The model under review builds one solid part; all positions refer to its coordinate system, in mm. A direction names the side the tool comes from. Give positions to 0.01 mm unless a question says otherwise; leave off trailing zeros. Order: outer loops, then holes, each group sorted by start corner. A loop starts at its lowest first (then second) coordinate and runs counter-clockwise, first axis right, second up. Notation, with made-up numbers: (-11, -39) - (17, -39) arc R21 cw to (17, -5) - close; hole circle Ø6 at (32.5, 41). An arc over 180 degrees is marked (long way). Use a Markdown table: item, result. Add a question column.
```python
from build123d import *

# Parameters (mm, degrees)
SKETCH1_W           = 88.9
SKETCH1_H           = 25.4
SKETCH1_R           = 2.25
BOSS_EXTRUDE1_DEPTH = 3.175
SKETCH2_W           = 88.9
SKETCH2_H           = 28.575
SKETCH2_R           = 2.25
BOSS_EXTRUDE2_DEPTH = 3.175
FILLET1_R           = 1.5875
BOSS_EXTRUDE3_DEPTH = 19.05
SKETCH5_R           = 2.25
CUT_EXTRUDE1_DEPTH  = 100
FILLET2_R           = 6.35
BOSS_EXTRUDE4_START = 5
SKETCH6_R           = 3.175
SKETCH6_R_2         = 2.25
BOSS_EXTRUDE4_DEPTH = 5
FILLET3_R           = 2
FILLET4_R           = 6
FILLET5_R           = 2


with BuildPart() as part:
    # Sketch1 → Boss-Extrude1 (new body)
    with BuildSketch(Plane.XY):
        Rectangle(SKETCH1_W, SKETCH1_H)
        Circle(SKETCH1_R, mode=Mode.SUBTRACT)
        with Locations((-38.1, 0)):
            Circle(SKETCH1_R, mode=Mode.SUBTRACT)
        with Locations((38.1, 0)):
            Circle(SKETCH1_R, mode=Mode.SUBTRACT)
    extrude(amount=BOSS_EXTRUDE1_DEPTH)

    # Sketch2 → Boss-Extrude2 (add)
    with BuildSketch(Plane(origin=(0, 12.7, 0), x_dir=(1, 0, 0), z_dir=(0, 1, 0))):
        with Locations((0, 11.1125)):
            Rectangle(SKETCH2_W, SKETCH2_H)
        with Locations(Location((0, 12.7, 0), (0, 0, 180))):
            Circle(SKETCH2_R, mode=Mode.SUBTRACT)
        with Locations(Location((-38.1, 12.7, 0), (0, 0, 180))):
            Circle(SKETCH2_R, mode=Mode.SUBTRACT)
        with Locations(Location((38.1, 12.7, 0), (0, 0, 180))):
            Circle(SKETCH2_R, mode=Mode.SUBTRACT)
    extrude(amount=BOSS_EXTRUDE2_DEPTH)

    # Fillet1
    fillet1_edges = [part.edges().sort_by_distance(p)[0] for p in [
        (0, 15.875, 3.175),
    ]]
    fillet(fillet1_edges, radius=FILLET1_R)

    # Sketch4 → Boss-Extrude3 (add)
    with BuildSketch(Plane(origin=(0, 15.875, 0), x_dir=(1, 0, 0), z_dir=(0, 1, 0))):
        Polygon((-11, 12.7), (-11, 25.4), (-17.35, 25.4), (-17.35, 12.7), (-17.35, -1.5875), (-11, -1.5875), align=None)
        Polygon((11, 25.4), (11, 12.7), (11, -1.5875), (17.35, -1.5875), (17.35, 12.7), (17.35, 25.4), align=None)
    extrude(amount=BOSS_EXTRUDE3_DEPTH)

    # Sketch5 → Cut-Extrude1 (cut)
    with BuildSketch(Plane(origin=(17.35, 0, 0), x_dir=(0, 0, -1), z_dir=(1, 0, 0))):
        with Locations(Location((11.90625, 28.575, 0), (0, 0, 90))):
            Circle(SKETCH5_R)
    extrude(amount=-CUT_EXTRUDE1_DEPTH, mode=Mode.SUBTRACT)

    # Fillet2
    fillet2_edges = [part.edges().sort_by_distance(p)[0] for p in [
        (-14.175, 34.925, -25.4),
        (-14.175, 34.925, 1.5875),
        (14.175, 34.925, -25.4),
        (14.175, 34.925, 1.5875),
    ]]
    fillet(fillet2_edges, radius=FILLET2_R)

    # Sketch6 → Boss-Extrude4 (add)
    with BuildSketch(Plane(origin=(-11, 0, 0), x_dir=(0, 0, -1), z_dir=(1, 0, 0)).offset(BOSS_EXTRUDE4_START)):
        with Locations((11.90625, 28.575)):
            Circle(SKETCH6_R)
        with Locations(Location((11.90625, 28.575, 0), (0, 0, 90))):
            Circle(SKETCH6_R_2, mode=Mode.SUBTRACT)
    extrude(amount=-BOSS_EXTRUDE4_DEPTH)

    # Fillet3
    fillet3_edges = [part.edges().sort_by_distance(p)[0] for p in [
        (-11, 28.575, -8.73125),
    ]]
    fillet(fillet3_edges, radius=FILLET3_R)

    # Mirror2: part across plane


with BuildPart() as part_1:
    add(part.part)
    add(part.part.mirror(Plane(origin=(0, 0, 0), x_dir=(0, 0, 1), z_dir=(1, 0, 0))))

    # Fillet4
    # the kernel refuses this fillet: 6 mm, written as the material it adds along each edge
    with BuildSketch(Plane(origin=(-17.35, 15.875, -25.4), x_dir=(0, 1, 0), z_dir=(0, 0, 1))) as fillet4_piece_1:
        with BuildLine():
            CenterArc((FILLET4_R, FILLET4_R), FILLET4_R, 180, 90)
            Line((0, FILLET4_R), (0, 0))
            Line((0, 0), (FILLET4_R, 0))
        make_face()
    extrude(amount=26.9875)
    with BuildSketch(Plane(origin=(17.35, 15.875, 1.5875), x_dir=(1, 0, 0), z_dir=(0, 0, -1))) as fillet4_piece_2:
        with BuildLine():
            CenterArc((FILLET4_R, -FILLET4_R), FILLET4_R, 90, 90)
            Line((0, -FILLET4_R), (0, 0))
            Line((0, 0), (FILLET4_R, 0))
        make_face()
    extrude(amount=26.9875)

    # Fillet5
    # the kernel refuses this fillet: 2 mm, written as the material it adds along each edge
    with BuildSketch(Plane(origin=(-11, 15.875, 1.5875), x_dir=(0, 1, 0), z_dir=(0, 0, -1))) as fillet5_piece_1:
        with BuildLine():
            CenterArc((FILLET5_R, FILLET5_R), FILLET5_R, 180, 90)
            Line((0, FILLET5_R), (0, 0))
            Line((0, 0), (FILLET5_R, 0))
        make_face()
    extrude(amount=26.9875)
    with BuildSketch(Plane(origin=(11, 15.875, -25.4), x_dir=(-1, 0, 0), z_dir=(0, 0, 1))) as fillet5_piece_2:
        with BuildLine():
            CenterArc((FILLET5_R, -FILLET5_R), FILLET5_R, 90, 90)
            Line((0, -FILLET5_R), (0, 0))
            Line((0, 0), (FILLET5_R, 0))
        make_face()
    extrude(amount=26.9875)


solid = part_1.part
```
Q1. We need section D-D (x = 38.5). Write out the cut boundary in (y, z) (1 decimal).
Q2. We need section B-B (x = 0). Count the separate pieces of the cut face and the enclosed holes in it, plus the area to 3 significant figures.
Q3. Draft analysis for pull direction Z (two halves, no side actions). For faces 1 (the cylindrical face through (14.219, 33.015, -0.223)), 2 (the cylindrical face through (-35.852, 14.265, -12.601)), 3 (the flat face through (-1, 12.7, -10)), state which applies: pulls with the +Z half, pulls with the -Z half, needs draft (parallel to the pull), parting line crosses it, or undercut.
Q4. Machinability: for faces 4 (the cylindrical face through (-7.479, 25.758, -13.371)), 5 (the flat face through (34, 15.875, -12)), 6 (the flat face through (14, 22, 1.588)), which of the approach directions +Z, -Z, +X, -X, +Y, -Y give a long, thin tool a straight path to every point of the face, cutting with its end or side? Answer none if there is none.
Q5. Clearance check with flat-ended pins moving along their axes: P1, Ø4, axis at y = 25.5, z = -18, coming from the -X side; P2, Ø4, axis at x = -17, y = 21.5, coming from the +Z side; P3, Ø4, axis at x = 0, z = -12.7, coming from the +Y side; P4, Ø1.5, axis at y = 18.5, z = -14, coming from the -X side. State where each tip first meets the part, or that it passes through.
Q6. We need section A-A (y = 0). Write out the cut boundary in (x, z) (3 decimals), plus the area to 3 significant figures.
Q7. Wall thickness on probe 1 along X at (y, z) = (13.95, -12.7); probe 2 along X at (y, z) = (31, -1); probe 3 along Y at (x, z) = (0, 0.75) (3 decimals): over which ranges is each line inside the solid? List them lowest first.
Q8. We need section C-C (z = -1.5). Write out the cut boundary in (x, y) (3 decimals), plus the area to 3 significant figures.
Here are the results:
| question | item | result |
|---|---|---|
| 1 | outline | (-12.7, 0) - (-2.2, 0) - (-2.2, 3.2) - (-12.7, 3.2) - close; (2.2, 0) - (12.7, 0) - (12.7, -10.5) - (15.9, -10.5) - (15.9, 1.6) arc R1.6 ccw to (14.3, 3.2) - (2.2, 3.2) - close; (12.7, -25.4) - (15.9, -25.4) - (15.9, -14.9) - (12.7, -14.9) - close |
| 2 | separate pieces | 3 |
| 2 | enclosed holes | 0 |
| 2 | area | 142 mm2 |
| 3 | face 1 | pulls with the +Z half |
| 3 | face 2 | undercut |
| 3 | face 3 | needs draft |
| 4 | face 4 | none |
| 4 | face 5 | +Z, -Z, +X, +Y |
| 4 | face 6 | +Z, +X, -X, +Y |
| 5 | P1 | x = -17.35 |
| 5 | P2 | z = 1.59 |
| 5 | P3 | through |
| 5 | P4 | x = -18.99 |
| 6 | outline | (-44.45, 0) - (-40.35, 0) - (-40.35, 3.175) - (-44.45, 3.175) - close; (-35.85, 0) - (-2.25, 0) - (-2.25, 3.175) - (-35.85, 3.175) - close; (2.25, 0) - (35.85, 0) - (35.85, 3.175) - (2.25, 3.175) - close; (40.35, 0) - (44.45, 0) - (44.45, 3.175) - (40.35, 3.175) - close |
| 6 | area | 239 mm2 |
| 7 | probe 1 | -44.45 to -40.35, -35.85 to -2.25, 2.25 to 35.85, 40.35 to 44.45 |
| 7 | probe 2 | -17.35 to -11, 11 to 17.35 |
| 7 | probe 3 | -12.7 to -2.25, 2.25 to 15.875 |
| 8 | outline | (-44.45, 12.7) - (44.45, 12.7) - (44.45, 15.875) - (23.35, 15.875) arc R6 cw to (17.35, 21.875) - (17.35, 34.023) - (11, 34.023) - (11, 17.875) arc R2 cw to (9, 15.875) - (-9, 15.875) arc R2 cw to (-11, 17.875) - (-11, 34.023) - (-17.35, 34.023) - (-17.35, 21.875) arc R6 cw to (-23.35, 15.875) - (-44.45, 15.875) - close |
| 8 | area | 530 mm2 |
